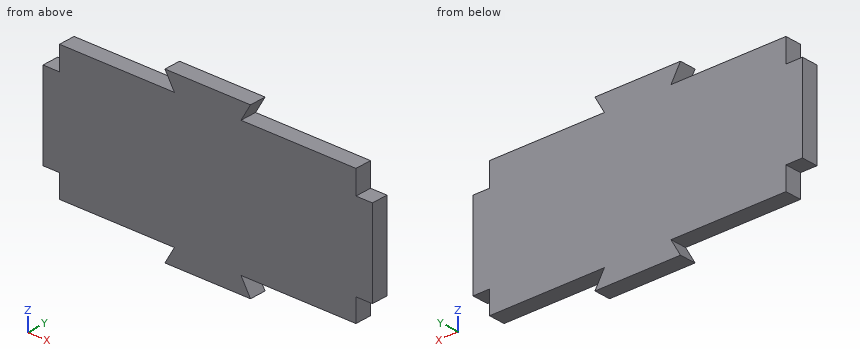
from build123d import *

# Parameters (mm, degrees)
BOSS_EXTRUDE1_DEPTH = 5


with BuildPart() as part:
    # Sketch2 → Boss-Extrude1 (new body)
    with BuildSketch(Plane(origin=(0, 0, 0), x_dir=(-1, 0, 0), z_dir=(0, 1, 0))):
        Polygon((45, 20), (10.103629711, 20), (12.990381057, 25), (-12.990381057, 25), (-10.103629711, 20), (-45, 20), (-45, 12.876959441), (-50, 12.876959441), (-50, -13.103802672), (-45, -13.103802672), (-45, -20), (-10.103629711, -20), (-12.990381057, -25), (12.990381057, -25), (10.103629711, -20), (45, -20), (45, -13.103802672), (50, -13.103802672), (50, 12.876959441), (45, 12.876959441), align=None)
    extrude(amount=BOSS_EXTRUDE1_DEPTH)


solid = part.part
Part model, mm, in its own coordinate system. Coordinates: 2 decimals unless noted, no trailing zeros. Order: outer loops, then holes, each group sorted by start corner. A loop starts at its lowest first (then second) coordinate and runs counter-clockwise, first axis right, second up.
(1) Slice it at B-B, the plane x = 17.5. Write the cut outline in (y, z), and give its area (3 significant figures).
Check sheet entries:
outline: (0, -20) - (5, -20) - (5, 20) - (0, 20) - close
area: 200 mm2
(2) Slice it at A-A, the plane y = 1. Write the cut outline in (x, z), and give its area (3 significant figures).
Check sheet entries:
outline: (-50, -13.1) - (-45, -13.1) - (-45, -20) - (-10.1, -20) - (-12.99, -25) - (12.99, -25) - (10.1, -20) - (45, -20) - (45, -13.1) - (50, -13.1) - (50, 12.88) - (45, 12.88) - (45, 20) - (10.1, 20) - (12.99, 25) - (-12.99, 25) - (-10.1, 20) - (-45, 20) - (-45, 12.88) - (-50, 12.88) - close
area: 4,090 mm2
(3) Slice it at C-C, the plane z = 16.5. Write the cut outline in (x, y), and give its area (3 significant figures).
Check sheet entries:
outline: (-45, 0) - (45, 0) - (45, 5) - (-45, 5) - close
area: 450 mm2
(4) Probe L1, parallel to Z at x = 40, y = 1.25; L2, parallel to X at y = 1.75, z = 18; L3, parallel to X at y = 0.25, z = 21. List the from-to ranges inside material, lowest first.
Check sheet entries:
L1: z = -20 to 20
L2: x = -45 to 45
L3: x = -10.68 to 10.68
(5) Pin check, flat tips, straight feed: pin 1 Ø2.5 at (y, z) = (3.5, 15) entering from -X; pin 2 Ø2.5 at (x, y) = (34, 2.5) entering from -Z; pin 3 Ø4 at (x, z) = (4, 2.5) entering from -Y; pin 4 Ø3 at (y, z) = (0.5, 18) entering from +X. Stop position of each tip, or through.
Check sheet entries:
pin 1: stops at x = -45
pin 2: stops at z = -20
pin 3: stops at y = 0
pin 4: stops at x = 45
